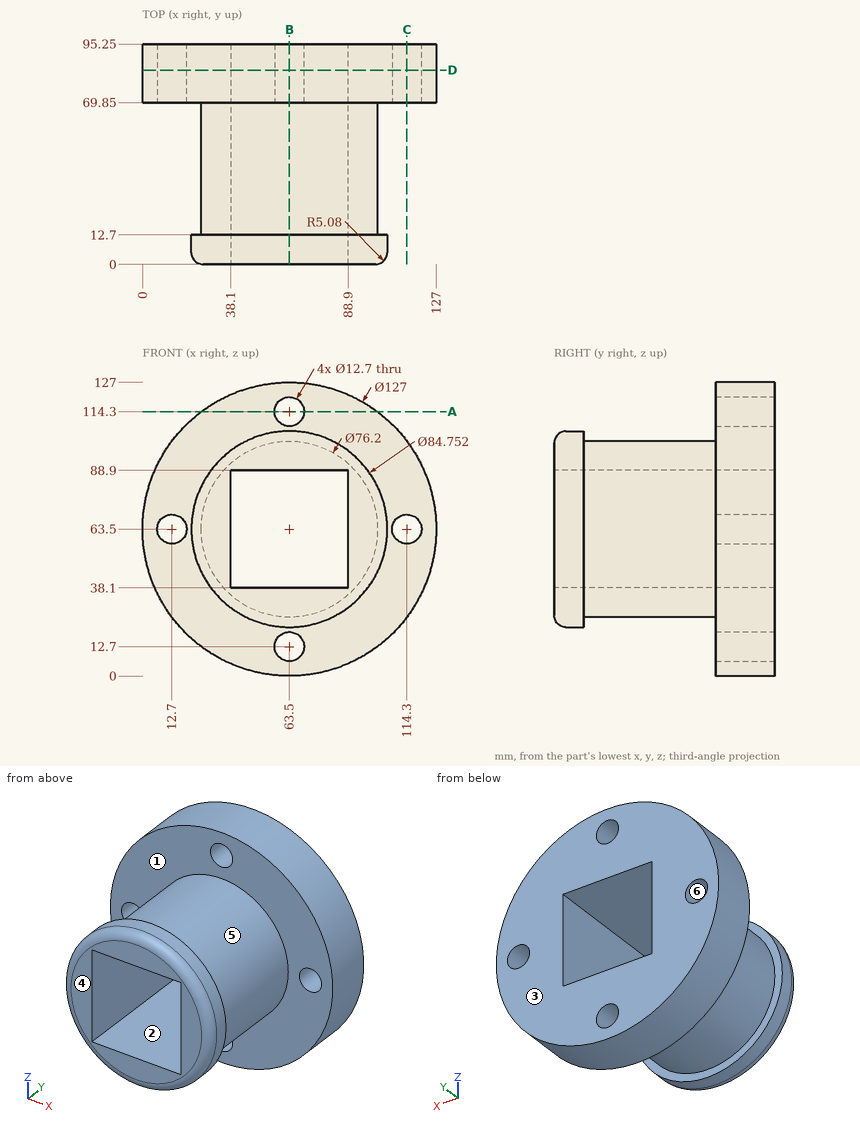
Can you work these out from the drawing? Everything is in mm from the part's minimum corner. A direction names the side the tool comes from. Give positions to 0.01 mm unless a question says otherwise; leave off trailing zeros. Order: outer loops, then holes, each group sorted by start corner. A loop starts at its lowest first (then second) coordinate and runs counter-clockwise, first axis right, second up.
Item 1: I need wall thicknesses on line 1 (Z direction, x = 63.5, y = 76); line 2 (X direction, y = 79, z = 63); line 3 (X direction, y = 32, z = 63). Which ranges of each line are inside material? Lowest first, please.
Item 2: I'm going to push flat-ended pins straight in: pin 1 (12 mm diameter, centred on y = 72, z = 112, fed in from +X); pin 2 (10 mm diameter, centred on x = 72.5, y = 72, fed in from -Z); pin 3 (8 mm diameter, centred on x = 25.5, z = 22, fed in from -Y). Where does each tip first touch, or does it pass through?
Item 3: For the marked faces 1, 2 and 3, which set-ups out of +Z, -Z, +X, -X, +Y, -Y let a thin tool reach every point of the face, with its end or its side?
Item 4: If we section it at D-D, the plane y = 84: Write out the boundary of the cut face in (x, z), plus the area to 3 significant figures.
Item 5: If we section it at B-B, the plane x = 63.5: Write out the boundary of the cut face in (y, z), plus the area to 3 significant figures.
Item 6: If we section it at C-C, the plane x = 114.3: Write out the boundary of the cut face in (y, z), plus the area to 3 significant figures.
Item 7: If we mould it in two halves opening along Z, with no side actions, what happens to the marked faces 4, 5 and 6? For each: pulls with the +Z half, pulls with the -Z half, needs draft (parallel to the pull), parting line crosses it, or undercut.
Item 8: If we section it at A-A, the plane z = 114.3: Write out the boundary of the cut face in (x, y).
Values:
1. line 1: z = 0 to 6.35, 19.05 to 38.1, 88.9 to 107.95, 120.65 to 127
1. line 2: x = 0 to 6.37, 19.03 to 38.1, 88.9 to 107.97, 120.63 to 127
1. line 3: x = 25.4 to 38.1, 88.9 to 101.6
2. pin 1: stops at x = 110.68
2. pin 2: stops at z = 0.13
2. pin 3: stops at y = 69.85
3. face 1: none
3. face 2: +Y, -Y
3. face 3: +Z, -Z, +X, -X, +Y
4. outline: circle Ø127 at (63.5, 63.5); hole circle Ø12.7 at (12.7, 63.5); hole (38.1, 38.1) - (88.9, 38.1) - (88.9, 88.9) - (38.1, 88.9) - close; hole circle Ø12.7 at (63.5, 12.7); hole circle Ø12.7 at (63.5, 114.3); hole circle Ø12.7 at (114.3, 63.5)
4. area: 9,580 mm2
5. outline: (0, 26.2) arc R5.08 ccw to (5.08, 21.12) - (12.7, 21.12) - (12.7, 25.4) - (69.85, 25.4) - (69.85, 19.05) - (95.25, 19.05) - (95.25, 38.1) - (0, 38.1) - close; (0, 88.9) - (95.25, 88.9) - (95.25, 107.95) - (69.85, 107.95) - (69.85, 101.6) - (12.7, 101.6) - (12.7, 105.88) - (5.08, 105.88) arc R5.08 ccw to (0, 100.8) - close; (69.85, 0) - (95.25, 0) - (95.25, 6.35) - (69.85, 6.35) - close; (69.85, 120.65) - (95.25, 120.65) - (95.25, 127) - (69.85, 127) - close
5. area: 3,160 mm2
6. outline: (69.85, 25.4) - (95.25, 25.4) - (95.25, 57.15) - (69.85, 57.15) - close; (69.85, 69.85) - (95.25, 69.85) - (95.25, 101.6) - (69.85, 101.6) - close
6. area: 1,610 mm2
7. face 4: needs draft
7. face 5: parting line crosses it
7. face 6: undercut
8. outline: (25.4, 69.85) - (57.15, 69.85) - (57.15, 95.25) - (25.4, 95.25) - close; (69.85, 69.85) - (101.6, 69.85) - (101.6, 95.25) - (69.85, 95.25) - close
